```python
from build123d import *

# Parameters (mm, degrees)
ESBO_O1_W                = 18
ESBO_O1_H                = 35
RESSALTO_EXTRUS_O1_DEPTH = 1.5
CORTE_EXTRUS_O1_REACH    = 21.906
ESBO_O2_W                = 13
ESBO_O2_H                = 23
CORTE_EXTRUS_O2_REACH    = 21.906
ESBO_O3_R                = 0.85
FILETE1_R                = 2
ESBO_O4_W                = 3
ESBO_O4_H                = 10
RESSALTO_EXTRUS_O2_DEPTH = 83.68
RESSALTO_EXTRUS_O2_TAPER = -2
ESBO_O5_W                = 22.844339982
ESBO_O5_H                = 15.844339982
RESSALTO_EXTRUS_O3_DEPTH = 2
CORTE_EXTRUS_O3_REACH    = 121.568
ESBO_O6_R                = 1.75


with BuildPart() as part:
    # Esboço1 → Ressalto-extrusão1 (new, symmetric)
    with BuildSketch(Plane(origin=(0, 0, 0), x_dir=(0, 0, -1), z_dir=(1, 0, 0))):
        Rectangle(ESBO_O1_W, ESBO_O1_H)
    extrude(amount=RESSALTO_EXTRUS_O1_DEPTH, both=True)

    # Esboço2 → Corte-extrusão1 (cut, up to next)
    with BuildSketch(Plane(origin=(1.5, 0, 0), x_dir=(0, 0, -1), z_dir=(1, 0, 0)), mode=Mode.PRIVATE) as corte_extrus_o1_sk1:
        Rectangle(ESBO_O2_W, ESBO_O2_H)
    corte_extrus_o1_tool1 = extrude(corte_extrus_o1_sk1.sketch, amount=-CORTE_EXTRUS_O1_REACH, mode=Mode.PRIVATE) & part.part
    add(corte_extrus_o1_tool1.solids().sort_by_distance((1.5, 0, 0))[0], mode=Mode.SUBTRACT)

    # Esboço3 → Corte-extrusão2 (cut, up to next)
    with BuildSketch(Plane.ZY.offset(1.5), mode=Mode.PRIVATE) as corte_extrus_o2_sk1:
        with Locations((0, 14)):
            Circle(ESBO_O3_R)
    corte_extrus_o2_tool1 = extrude(corte_extrus_o2_sk1.sketch, amount=-CORTE_EXTRUS_O2_REACH, mode=Mode.PRIVATE) & part.part
    # Esboço3 → Corte-extrusão2 (cut, up to next)
    with BuildSketch(Plane.ZY.offset(1.5), mode=Mode.PRIVATE) as corte_extrus_o2_sk2:
        with Locations((0, -14)):
            Circle(ESBO_O3_R)
    corte_extrus_o2_tool2 = extrude(corte_extrus_o2_sk2.sketch, amount=-CORTE_EXTRUS_O2_REACH, mode=Mode.PRIVATE) & part.part
    add(corte_extrus_o2_tool1.solids().sort_by_distance((-1.5, 14, 0))[0], mode=Mode.SUBTRACT)
    add(corte_extrus_o2_tool2.solids().sort_by_distance((-1.5, -14, 0))[0], mode=Mode.SUBTRACT)

    # Filete1
    filete1_edges = [part.edges().sort_by_distance(p)[0] for p in [
        (0, -17.5, -9),
        (0, -17.5, 9),
        (0, 17.5, 9),
        (0, 17.5, -9),
    ]]
    fillet(filete1_edges, radius=FILETE1_R)

    # Esboço4 → Ressalto-extrusão2 (add)
    with BuildSketch(Plane.XZ.offset(17.5)):
        Rectangle(ESBO_O4_W, ESBO_O4_H)
    extrude(amount=RESSALTO_EXTRUS_O2_DEPTH, taper=RESSALTO_EXTRUS_O2_TAPER)

    # Esboço5 → Ressalto-extrusão3 (add)
    with BuildSketch(Plane.XZ.offset(101.18)):
        Rectangle(ESBO_O5_W, ESBO_O5_H)
    extrude(amount=RESSALTO_EXTRUS_O3_DEPTH)

    # Esboço6 → Corte-extrusão3 (cut, up to next)
    with BuildSketch(Plane(origin=(0, -101.18, 0), x_dir=(1, 0, 0), z_dir=(0, 1, 0)), mode=Mode.PRIVATE) as corte_extrus_o3_sk1:
        with Locations(Location((7.922169991, 0, 0), (0, 0, 270))):
            Circle(ESBO_O6_R)
    corte_extrus_o3_tool1 = extrude(corte_extrus_o3_sk1.sketch, amount=-CORTE_EXTRUS_O3_REACH, mode=Mode.PRIVATE) & part.part
    # Esboço6 → Corte-extrusão3 (cut, up to next)
    with BuildSketch(Plane(origin=(0, -101.18, 0), x_dir=(1, 0, 0), z_dir=(0, 1, 0)), mode=Mode.PRIVATE) as corte_extrus_o3_sk2:
        with Locations(Location((-7.922169991, 0, 0), (0, 0, 270))):
            Circle(ESBO_O6_R)
    corte_extrus_o3_tool2 = extrude(corte_extrus_o3_sk2.sketch, amount=-CORTE_EXTRUS_O3_REACH, mode=Mode.PRIVATE) & part.part
    add(corte_extrus_o3_tool1.solids().sort_by_distance((7.92217, -101.18, 0))[0], mode=Mode.SUBTRACT)
    add(corte_extrus_o3_tool2.solids().sort_by_distance((-7.92217, -101.18, 0))[0], mode=Mode.SUBTRACT)


solid = part.part
```
Could you check a few things on this model? Use its own coordinates, in mm. A direction names the side the tool comes from. Round coordinates to 2 decimals unless told otherwise and drop trailing zeros. Write each loop counter-clockwise with the first axis right and the second up, starting at its lowest first coordinate (ties: lowest second). Pieces come first, ordered by that corner, then holes. Notation, with made-up numbers: M 35,72 L 39,72 A13 ccw 39,96 Z; hole C 9.25,-38.75 d2. An arc over 180 degrees is marked long. Write each question's results on one line, items separated by ' | '. Start each with the question number.
1. I need wall thicknesses on L1, parallel to Y at x = -0.2, z = 0; L2, parallel to X at y = -101.7, z = 0; L3, parallel to Y at x = 0.25, z = -0.5. Which ranges of each line are inside material? Lowest first, please. Write a range as from..to.
2. On a 3-axis mill with a long thin cutter (end or side, diameter ignored), from which of +Z, -Z, +X, -X, +Y, -Y can I reach the whole of each face in a straight line? I mean faces 1 (the face through (-1.5, 4, 8)), 2 (the face through (8, -101.18, 2)), 3 (the face through (0, 11.5, 0)), 4 (the face through (0, -17.5, -6)). Say none if no direction works.
3. Imagine slicing it at A-A on y = 0. List the corners of the cut face in (x, z) for me, and give its area (3 significant figures).
4. Imagine slicing it at B-B on x = 0.5. Count the separate pieces of the cut face and the enclosed holes in it, and give its area (3 significant figures).
5. I'm going to push flat-ended pins straight in: pin 1 Ø1.5 at (y, z) = (-13.5, -5.5) entering from -X; pin 2 Ø6 at (y, z) = (-73.5, -6) entering from -X; pin 3 Ø2 at (y, z) = (-32, -4) entering from +X. Where does each tip first touch, or does it pass through?
6. Thinking about a two-plate mould opening in Z: for faces 5 (the face through (1.5, 4, 8)), 6 (the face through (0, -11.5, 0)), 7 (the face through (0.02, -16.93, -8.4)), which applies, +Z half, -Z half, draft (parallel to the pull), parting line (faces both ways), or undercut?
Result sheet:
1) L1: y = -103.18..-14.85, -13.15..-11.5, 11.5..13.15, 14.85..17.5 | L2: x = -11.42..-9.67, -6.17..6.17, 9.67..11.42 | L3: y = -103.18..-14.69, -13.31..-11.5, 11.5..13.31, 14.69..17.5
2) face 1: +Z, -Z, -X, +Y | face 2: +Z, -Z, +X, +Y | face 3: +X, -X | face 4: -Z, +X, -X
3) outline: M -1.5,-9 L 1.5,-9 L 1.5,-6.5 L -1.5,-6.5 Z; M -1.5,6.5 L 1.5,6.5 L 1.5,9 L -1.5,9 Z | area: 15.0 mm^2
4) separate pieces: 1 | enclosed holes: 3 | area: 1,440 mm^2
5) pin 1: stops at x = -1.5 | pin 2: stops at x = -3.56 | pin 3: stops at x = 2.04
6) face 5: draft | face 6: undercut | face 7: -Z half
